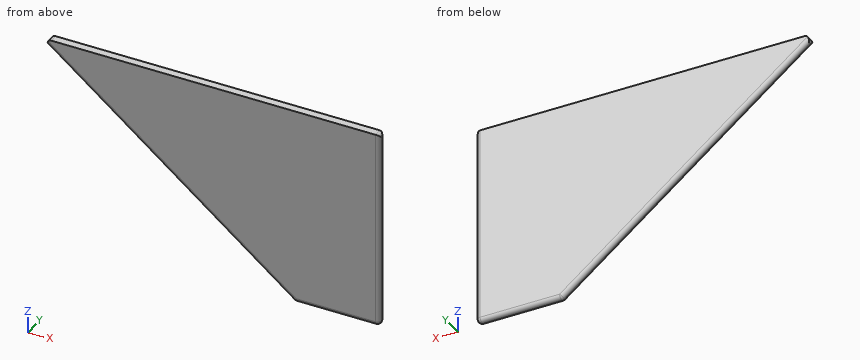
from build123d import *

# Parameters (mm, degrees)
BOSS_EXTRUDE1_DEPTH = 4.76
FILLET3_R           = 2.38


with BuildPart() as part:
    # Sketch1 → Boss-Extrude1 (new body)
    with BuildSketch(Plane(origin=(0, 0, 0), x_dir=(1, 0, 0), z_dir=(0, 1, 0))):
        Polygon((0, 0), (0, 120), (-50, 120), (-200, 0), align=None)
    extrude(amount=BOSS_EXTRUDE1_DEPTH)

    # Fillet3
    fillet3_edges = [part.edges().sort_by_distance(p)[0] for p in [
        (-25, 4.76, -120),
        (-125, 4.76, -60),
        (-125, 0, -60),
        (-25, 0, -120),
        (0, 0, -60),
        (-200, 2.38, 0),
        (-50, 2.38, -120),
        (0, 2.38, -120),
        (0, 2.38, 0),
        (0, 4.76, -60),
    ]]
    fillet(fillet3_edges, radius=FILLET3_R - 0.0001)  # a hair under: the kernel refuses the full size


solid = part.part
The listing builds one solid part. Answer for the finished solid, in the listing's coordinates (mm). Give positions to 0.01 mm unless a question says otherwise; leave off trailing zeros. Loops run counter-clockwise (first coordinate to the right, second up) from the corner with the lowest first, then second, coordinate; pieces in that order, holes last. Notation, with made-up numbers: (58.25, 47.5) - (109.25, 47.5) arc R17 cw to (109.25, 72.5) - close; hole circle Ø7 at (-15, 2.5). An arc over 180 degrees is marked (long way). Answer as a JSON object with one key per item and string values.
1. Flat-ended cylindrical pins translate along their axes: pin 1 Ø1.5 at (x, y) = (-174, 1) entering from -Z; pin 2 Ø1 at (y, z) = (3.5, -96.5) entering from -X; pin 3 Ø2 at (y, z) = (3, -37) entering from -X. Find the tip coordinate at first contact, or state that the pin passes through.
Determined:
{"pin 1": "z = -21.04", "pin 2": "x = -79.65", "pin 3": "x = -154.92"}
2. A cutting plane is placed at A-A (y = 3.4). Write down the section's boundary in (x, z).
Determined:
{"outline": "(-195.36, -3.42) - (-50.51, -119.3) arc R2.15 ccw to (-49.17, -119.77) - (-2.38, -119.77) arc R2.15 ccw to (-0.23, -117.62) - (-0.23, -1.36) arc R2.38 ccw to (-2.38, 0) - (-193.22, 0) arc R2.38 ccw to start"}
3. Find the intervals of material crossed by L1, parallel to Z at x = -43, y = 2.65; L2, parallel to X at y = 0.8, z = -33.5; L3, parallel to Z at x = -54, y = 2.5, in increasing order. Write a range as [from, to].
Determined:
{"L1": "[-119.98, 0]", "L2": "[-157.16, -0.6]", "L3": "[-116.8, 0]"}
